Here's how the part is built. I have some questions about the finished solid (model axes, mm). Coordinates: 2 decimals unless noted, no trailing zeros. Write each loop counter-clockwise with the first axis right and the second up, starting at its lowest first coordinate (ties: lowest second). Pieces come first, ordered by that corner, then holes.
```python
from build123d import *

# Parameters (mm, degrees)
EXTRUDE_1_DEPTH = 0.3


with BuildPart() as part:
    # Эскиз1 → Бобышка-Вытянуть1 (new body)
    with BuildSketch(Plane(origin=(0, 0, 0), x_dir=(1, 0, 0), z_dir=(0, 1, 0))):
        with BuildLine():
            Line((-11.404541059, 16.350155755), (-11.404541059, 28.750155755))
            Line((-11.404541059, 28.750155755), (-18.590239448, 28.750155755))
            ThreePointArc((-18.590239448, 28.750155755), (-23.404541059, 25.100155755), (-28.218842669, 28.750155755))
            Line((-28.218842669, 28.750155755), (-35.404541059, 28.750155755))
            Line((-35.404541059, 28.750155755), (-35.404541059, 16.350155755))
            Line((-35.404541059, 16.350155755), (-31.404541059, 16.350155755))
            Line((-31.404541059, 16.350155755), (-31.404541059, 14.350155755))
            Line((-31.404541059, 14.350155755), (-34.604541059, 14.350155755))
            ThreePointArc((-34.604541059, 14.350155755), (-34.958094449, 14.203709145), (-35.104541059, 13.850155755))
            Line((-35.104541059, 13.850155755), (-35.104541059, -3.649844245))
            ThreePointArc((-35.104541059, -3.649844245), (-34.958094449, -4.003397636), (-34.604541059, -4.149844245))
            Line((-34.604541059, -4.149844245), (-31.404541059, -4.149844245))
            Line((-31.404541059, -4.149844245), (-31.404541059, -6.149844245))
            Line((-31.404541059, -6.149844245), (-35.404541059, -6.149844245))
            Line((-35.404541059, -6.149844245), (-35.404541059, -18.549844245))
            Line((-35.404541059, -18.549844245), (-28.218842669, -18.549844245))
            ThreePointArc((-28.218842669, -18.549844245), (-23.404541059, -14.899844245), (-18.590239448, -18.549844245))
            Line((-18.590239448, -18.549844245), (-11.404541059, -18.549844245))
            Line((-11.404541059, -18.549844245), (-11.404541059, -6.149844245))
            Line((-11.404541059, -6.149844245), (-15.404541059, -6.149844245))
            Line((-15.404541059, -6.149844245), (-15.404541059, -4.149844245))
            Line((-15.404541059, -4.149844245), (-10.604541059, -4.149844245))
            ThreePointArc((-10.604541059, -4.149844245), (-10.250987668, -4.003397636), (-10.104541059, -3.649844245))
            Line((-10.104541059, -3.649844245), (-10.104541059, 13.850155755))
            ThreePointArc((-10.104541059, 13.850155755), (-10.250987668, 14.203709145), (-10.604541059, 14.350155755))
            Line((-10.604541059, 14.350155755), (-15.404541059, 14.350155755))
            Line((-15.404541059, 14.350155755), (-15.404541059, 16.350155755))
            Line((-15.404541059, 16.350155755), (-11.404541059, 16.350155755))
        make_face()
        with BuildLine():
            Line((-17.404541059, 6.700155755), (-15.504541059, 6.700155755))
            ThreePointArc((-15.504541059, 6.700155755), (-13.904541059, 5.100155755), (-15.504541059, 3.500155755))
            Line((-15.504541059, 3.500155755), (-17.404541059, 3.500155755))
            ThreePointArc((-17.404541059, 3.500155755), (-19.004541059, 5.100155755), (-17.404541059, 6.700155755))
        make_face(mode=Mode.SUBTRACT)
    extrude(amount=EXTRUDE_1_DEPTH)


solid = part.part
```
1) Imagine slicing it at D-D on x = -18. Please give me the cut outline in (y, z).
Values follow:
outline: (0, -28.75) - (0.3, -28.75) - (0.3, -6.59) - (0, -6.59) - close; (0, -3.62) - (0.3, -3.62) - (0.3, 18.55) - (0, 18.55) - close
2) I need wall thicknesses on probe 1 along Z at (x, y) = (-33.75, 0.2); probe 2 along X at (y, z) = (0.2, -20); probe 3 along X at (y, z) = (0.2, -12.5). Which ranges of each line are inside material? Lowest first, please.
Values follow:
probe 1: z = -28.75 to -16.35, -14.35 to 4.15, 6.15 to 18.55
probe 2: x = -35.4 to -11.4
probe 3: x = -35.1 to -10.1
3) Imagine slicing it at A-A on x = -12.5. Please give me the cut outline in (y, z).
Values follow:
outline: (0, -28.75) - (0.3, -28.75) - (0.3, -16.35) - (0, -16.35) - close; (0, -14.35) - (0.3, -14.35) - (0.3, 4.15) - (0, 4.15) - close; (0, 6.15) - (0.3, 6.15) - (0.3, 18.55) - (0, 18.55) - close
4) Imagine slicing it at C-C on z = -5. Please give me the cut outline in (x, y), then the cut area to 3 significant figures.
Values follow:
outline: (-35.1, 0) - (-19, 0) - (-19, 0.3) - (-35.1, 0.3) - close; (-13.91, 0) - (-10.1, 0) - (-10.1, 0.3) - (-13.91, 0.3) - close
area: 5.97 mm2
